Source: CAD feature listing. Evaluate the final solid. Frame: model axes, mm. A direction names the side the tool comes from. Coordinates: 2 decimals unless noted, no trailing zeros. Order: outer loops, then holes, each group sorted by start corner. A loop starts at its lowest first (then second) coordinate and runs counter-clockwise, first axis right, second up. Notation, with made-up numbers: (-5, 66.5) -> (39, 66.5) arc R21 cw to (39, 88.5) -> close; hole circle Ø1 at (-17, 83.5). An arc over 180 degrees is marked (long way). Write each question's results on one line, items separated by ' | '. Start each with the question number.
from build123d import *

# Parameters (mm, degrees)
SKETCH1_W           = 25
SKETCH1_H           = 23.7
BOSS_EXTRUDE1_DEPTH = 3
BOSS_EXTRUDE2_DEPTH = 23.7
SKETCH4_W           = 10
SKETCH4_H           = 10
CUT_EXTRUDE1_DEPTH  = 1.5
CUT_EXTRUDE2_DEPTH  = 3
SKETCH6_W           = 10
SKETCH6_H           = 3
BOSS_EXTRUDE3_DEPTH = 1.5
CHAMFER1_SIZE       = 1.5
CHAMFER1_SIZE2      = 2.598076211
SKETCH7_W           = 20
SKETCH7_H           = 3
CUT_EXTRUDE3_DEPTH  = 1.5
FILLET1_R           = 1
SKETCH8_W           = 8
SKETCH8_H           = 2
CUT_EXTRUDE4_DEPTH  = 1
FILLET2_R           = 10
FILLET3_R           = 1
CHAMFER3_SIZE       = 1
CHAMFER4_SIZE       = 1
CHAMFER5_SIZE       = 1
CHAMFER5_SIZE2      = 1.191753593


with BuildPart() as part:
    # Sketch1 → Boss-Extrude1 (new body)
    with BuildSketch(Plane.XY):
        with Locations((12.5, 11.85)):
            Rectangle(SKETCH1_W, SKETCH1_H)
    extrude(amount=BOSS_EXTRUDE1_DEPTH)

    # Sketch2 → Boss-Extrude2 (add)
    with BuildSketch(Plane.XZ):
        Polygon((0, 0), (-2.5, 0), (0, 3), align=None)
        Polygon((25, 0), (27.5, 0), (25, 3), align=None)
    extrude(amount=-BOSS_EXTRUDE2_DEPTH)

    # Sketch4 → Cut-Extrude1 (cut)
    with BuildSketch(Plane(origin=(0, 0, 0), x_dir=(-1, 0, 0), z_dir=(0, 0, -1))):
        with Locations((-12.5, 12.7)):
            Rectangle(SKETCH4_W, SKETCH4_H)
    extrude(amount=-CUT_EXTRUDE1_DEPTH, mode=Mode.SUBTRACT)

    # Sketch5 → Cut-Extrude2 (cut)
    with BuildSketch(Plane(origin=(0, 0, 0), x_dir=(-1, 0, 0), z_dir=(0, 0, -1))):
        with BuildLine():
            Line((-17.5, 7.7), (-17.5, 23.7))
            Line((-17.5, 23.7), (-18.2, 23.7))
            Line((-18.2, 23.7), (-18.2, 7.7))
            ThreePointArc((-18.2, 7.7), (-17.85, 7.35), (-17.5, 7.7))
        make_face()
        with BuildLine():
            Line((-7.5, 7.7), (-7.5, 23.7))
            Line((-7.5, 23.7), (-6.8, 23.7))
            Line((-6.8, 23.7), (-6.8, 7.7))
            ThreePointArc((-6.8, 7.7), (-7.15, 7.35), (-7.5, 7.7))
        make_face()
    extrude(amount=-CUT_EXTRUDE2_DEPTH, mode=Mode.SUBTRACT)

    # Sketch6 → Boss-Extrude3 (add)
    with BuildSketch(Plane(origin=(0, 0, 0), x_dir=(-1, 0, 0), z_dir=(0, 0, -1))):
        with Locations((-12.5, 19.2)):
            Rectangle(SKETCH6_W, SKETCH6_H)
    extrude(amount=BOSS_EXTRUDE3_DEPTH)

    # Chamfer1
    chamfer1_edges = [part.edges().sort_by_distance(p)[0] for p in [
        (12.5, 17.7, -1.5),
    ]]
    chamfer1_side = [part.faces().sort_by_distance(p)[0] for p in [
        (12.5, 17.7, 0),
    ]]
    chamfer(chamfer1_edges, length=CHAMFER1_SIZE, length2=CHAMFER1_SIZE2, reference=chamfer1_side[0])

    # Sketch7 → Cut-Extrude3 (cut)
    with BuildSketch(Plane.XY.offset(3)):
        with Locations((12.5, 3.5)):
            Rectangle(SKETCH7_W, SKETCH7_H)
    extrude(amount=-CUT_EXTRUDE3_DEPTH, mode=Mode.SUBTRACT)

    # Fillet1
    fillet1_edges = [part.edges().sort_by_distance(p)[0] for p in [
        (12.5, 17.7, 1.5),
        (12.5, 7.7, 1.5),
    ]]
    fillet(fillet1_edges, radius=FILLET1_R)

    # Sketch8 → Cut-Extrude4 (cut)
    with BuildSketch(Plane(origin=(0, 0, 0), x_dir=(-1, 0, 0), z_dir=(0, 0, -1))):
        with Locations((-12.5, 21.7)):
            Rectangle(SKETCH8_W, SKETCH8_H)
    extrude(amount=-CUT_EXTRUDE4_DEPTH, mode=Mode.SUBTRACT)

    # Fillet2
    # the kernel refuses this fillet: 10 mm, written as the material it takes off along each edge
    with BuildSketch(Plane(origin=(25, 17.7, 0), x_dir=(0, -0.17402760364384265, 0.9847407746051655), z_dir=(-1, 0, 0))) as fillet2_piece_1_section:
        with BuildLine():
            CenterArc((5.512472708, 8.977269728), FILLET2_R, 221.911963519, 21.948914507)
            Line((-1.929248139, 2.297390175), (-2.673420224, 1.62940222))
            ThreePointArc((-2.673420224, 1.62940222), (-1.730420795, 0.505612375), (-0.765796725, -0.643082713))
            Line((-0.765796725, -0.643082713), (0.174027604, -0.984740775))
            Line((0.174027604, -0.984740775), (0.666397991, -0.897726973))
            Line((0.666397991, -0.897726973), (1.106950238, 0))
        make_face()
    fillet2_piece_1 = extrude(amount=25, mode=Mode.PRIVATE)
    fillet2_piece_1 = split(fillet2_piece_1, bisect_by=Plane(origin=(18.2, 17.7, 0), z_dir=(-1, 0, 0)), keep=Keep.TOP, mode=Mode.PRIVATE)
    fillet2_piece_1 = split(fillet2_piece_1, bisect_by=Plane(origin=(6.8, 17.7, 0), z_dir=(1, 0, 0)), keep=Keep.TOP, mode=Mode.PRIVATE)
    add(fillet2_piece_1, mode=Mode.SUBTRACT)

    # Fillet3
    # the kernel refuses this fillet: 1 mm, written as the material it takes off along each edge
    with BuildSketch(Plane(origin=(5.158770817, 7.7, 0), x_dir=(0, -1, 0), z_dir=(1, 0, 0))) as fillet3_piece_1_section:
        with BuildLine():
            CenterArc((0.936491673, -1), FILLET3_R, 90, 75.522487814)
            Line((-0.031754163, -0.75), (-0.128578747, -0.725))
            ThreePointArc((-0.128578747, -0.725), (-0.1, -0.5), (-0.1, 0))
            Line((-0.1, 0), (0, 0.1))
            Line((0, 0.1), (0.936491673, 0.1))
            Line((0.936491673, 0.1), (0.936491673, 0))
        make_face()
    fillet3_piece_1 = extrude(amount=14.682458366, mode=Mode.PRIVATE)
    fillet3_piece_1 = split(fillet3_piece_1, bisect_by=Plane(origin=(6.8, 7.7, 0), z_dir=(1, 0, 0)), keep=Keep.TOP, mode=Mode.PRIVATE)
    fillet3_piece_1 = split(fillet3_piece_1, bisect_by=Plane(origin=(18.2, 7.7, 0), z_dir=(-1, 0, 0)), keep=Keep.TOP, mode=Mode.PRIVATE)
    add(fillet3_piece_1, mode=Mode.SUBTRACT)

    # Chamfer3
    chamfer3_edges = [part.edges().sort_by_distance(p)[0] for p in [
        (-1.25, 0, 1.5),
        (26.25, 0, 1.5),
        (12.5, 0, 0),
    ]]
    chamfer(chamfer3_edges, length=CHAMFER3_SIZE)

    # Chamfer4
    chamfer4_edges = [part.edges().sort_by_distance(p)[0] for p in [
        (21.6, 23.7, 3),
        (12.5, 23.7, 3),
        (3.4, 23.7, 3),
    ]]
    chamfer(chamfer4_edges, length=CHAMFER4_SIZE)

    # Chamfer5
    chamfer5_edges = [part.edges().sort_by_distance(p)[0] for p in [
        (12.5, 20.7, 1),
    ]]
    chamfer5_side = [part.faces().sort_by_distance(p)[0] for p in [
        (12.5, 20.7, -0.315217391),
    ]]
    chamfer(chamfer5_edges, length=CHAMFER5_SIZE, length2=CHAMFER5_SIZE2, reference=chamfer5_side[0])


solid = part.part
(1) Section C-C on z = 2.6. Return the cut outline in (x, y).
(2) Section A-A on y = 15.5. Return the cut outline in (x, z).
(3) Reachability of faces 4 (the flat face through (12, 2, 2)), 5 (the flat face through (13, 20.7, -1)), 6 (the flat face through (12.556, 21.304, 0.507)), 7 (the flat face through (17.5, 17, 2)), 8 (the flat face through (12.4, 23.2, 2.5)) from +Z, -Z, +X, -X, +Y, -Y: full face, straight path, thin tool, end or side. Return the list, or none.
(4) Draft query along Y for faces 1 (the flat face through (13, 0, 2)), 2 (the flat face through (-1.267, 12.191, 1.479)), 3 (the flat face through (12, 4, 1.5)). Return one class per face: released by +Y, released by -Y, zero draft, split by the parting line, or undercut.
(5) Section D-D on y = 3.5. Return the cut outline in (x, z), then the cut area to 3 significant figures.
(6) Section B-B on x = 3. Return the cut outline in (y, z).
(7) First-contact query: P1, Ø0.8, axis at y = 3, z = 2.5, coming from the -X side; P2, Ø0.8, axis at y = 22, z = 0.5, coming from the -X side; P3, Ø2.5, axis at x = 14, y = 13.5, coming from the -Z side. Flat tips, straight axial feed; report the tip coordinate or a pass-through.
(8) Line query: L1, parallel to Y at x = 20, z = 1.9; L2, parallel to Y at x = 13.5, z = 0.3; L3, parallel to X at y = 14, z = 1.6. Output: solid intervals per line, ascending.
Results list:
1) outline: (-0.33, 1) -> (0.97, 0) -> (24.03, 0) -> (25.33, 1) -> (25.33, 23.1) -> (18.2, 23.1) -> (18.2, 7.7) arc R0.35 cw to (17.5, 7.7) -> (17.5, 23.1) -> (7.5, 23.1) -> (7.5, 7.7) arc R0.35 cw to (6.8, 7.7) -> (6.8, 23.1) -> (-0.33, 23.1) -> close; hole (2.5, 2) -> (22.5, 2) -> (22.5, 5) -> (2.5, 5) -> close
2) outline: (-2.5, 0) -> (6.8, 0) -> (6.8, 3) -> (0, 3) -> close; (7.5, 1.5) -> (17.5, 1.5) -> (17.5, 3) -> (7.5, 3) -> close; (18.2, 0) -> (27.5, 0) -> (25, 3) -> (18.2, 3) -> close
3) face 4: +Z | face 5: -Z, +X, -X, +Y | face 6: -Z | face 7: +Z, -Z, +Y | face 8: +Z, +X, -X, +Y
4) face 1: released by -Y | face 2: zero draft | face 3: undercut
5) outline: (-2.5, 0) -> (27.5, 0) -> (25, 3) -> (22.5, 3) -> (22.5, 1.5) -> (2.5, 1.5) -> (2.5, 3) -> (0, 3) -> close | area: 52.5 mm²
6) outline: (0, 1) -> (1, 0) -> (23.7, 0) -> (23.7, 2) -> (22.7, 3) -> (5, 3) -> (5, 1.5) -> (2, 1.5) -> (2, 3) -> (0, 3) -> close
7) P1: stops at x = -0.75 | P2: stops at x = -2.42 | P3: stops at z = 1.5
8) L1: y = 0 to 2, 5 to 23.7 | L2: y = 0.7 to 7.48, 18.15 to 21.06, 22.7 to 23.7 | L3: x = -1.17 to 6.8, 7.5 to 17.5, 18.2 to 26.17
